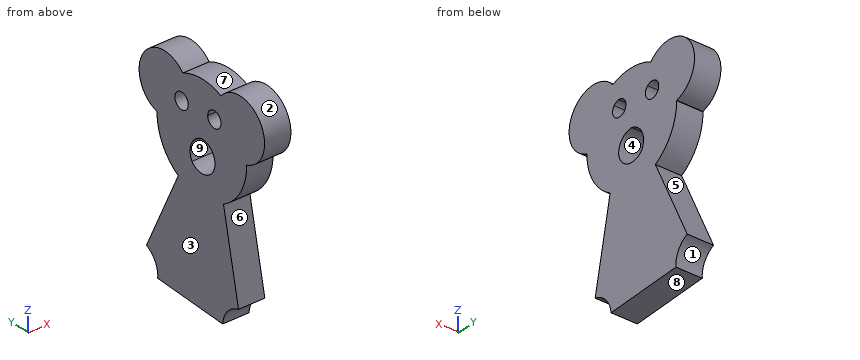
```python
from build123d import *

# Parameters (mm, degrees)
F1_DEPTH = 25


with BuildPart() as f1:
    # F0 (on Right) → F1 (new body)
    with BuildSketch(Plane.YZ):
        with BuildLine():
            Line((62.268494035, -117.2657224541), (26.5148173721, -42.9157082976))
            ThreePointArc((26.5148173721, -42.9157082976), (1.2487643575, -50.4304882639), (-24.3582585984, -44.1754320523))
            Line((-24.3582585984, -44.1754320523), (-41.1918519377, -124.9397814602))
            ThreePointArc((-41.1918519377, -124.9397814602), (-28.905337679, -132.0868997864), (-23.3544766233, -145.1722990748))
            Line((-23.3544766233, -145.1722990748), (49.5911414452, -139.3371221753))
            ThreePointArc((49.5911414452, -139.3371221753), (52.5088729266, -126.3365028199), (62.268494035, -117.2657224541))
        make_face()
        with BuildLine():
            ThreePointArc((26.5148173721, -42.9157082976), (44.0588165312, -24.5685621237), (50.4459469032, 0))
            ThreePointArc((50.4459469032, 0), (50.4457051903, 0.1561627636), (50.4449800541, 0.3123240306))
            ThreePointArc((50.4449800541, 0.3123240306), (48.3675580647, 14.3308368847), (42.4729821328, 27.2183641629))
            Line((42.4729821328, 27.2183641629), (27.7815824315, 27.2183641629))
            ThreePointArc((27.7815824315, 27.2183641629), (29.6215359729, 24.6926196845), (30.2725235865, 21.6363099275))
            ThreePointArc((30.2725235865, 21.6363099275), (19.7162138294, 14.7872975411), (17.7634647415, 27.2183641629))
            Line((17.7634647415, 27.2183641629), (-8.2927525458, 27.2183641629))
            ThreePointArc((-8.2927525458, 27.2183641629), (-7.0141543228, 24.9776791667), (-6.5704554783, 22.4362988324))
            ThreePointArc((-6.5704554783, 22.4362988324), (-16.6118358125, 15.379997677), (-19.8481584107, 27.2183641629))
            Line((-19.8481584107, 27.2183641629), (-42.4729821328, 27.2183641629))
            ThreePointArc((-42.4729821328, 27.2183641629), (-48.3583492389, 14.361880721), (-50.4445375277, 0.3770843017))
            ThreePointArc((-50.4445375277, 0.3770843017), (-43.5327032866, -25.4891605102), (-24.3582585984, -44.1754320523))
            ThreePointArc((-24.3582585984, -44.1754320523), (1.2487643575, -50.4304882639), (26.5148173721, -42.9157082976))
        make_face()
        with BuildLine():
            ThreePointArc((11.1447488889, -24.0004807711), (-13.3697300078, -20.7961057501), (0, 0))
            ThreePointArc((0, 0), (11.7053783119, -9.1523479333), (11.1447488889, -24.0004807711))
        make_face(mode=Mode.SUBTRACT)
        with BuildLine():
            Line((27.7815824315, 27.2183641629), (42.4729821328, 27.2183641629))
            ThreePointArc((42.4729821328, 27.2183641629), (33.2264505165, 37.9578258733), (21.3576968642, 45.7016667487))
            ThreePointArc((21.3576968642, 45.7016667487), (-0.0323808915, 50.4459365106), (-21.4163503965, 45.6742103889))
            ThreePointArc((-21.4163503965, 45.6742103889), (-33.2508085276, 37.9364902332), (-42.4729821328, 27.2183641629))
            Line((-42.4729821328, 27.2183641629), (-19.8481584107, 27.2183641629))
            ThreePointArc((-19.8481584107, 27.2183641629), (-17.5022305288, 29.105100824), (-14.6033657252, 29.9173419862))
            ThreePointArc((-14.6033657252, 29.9173419862), (-11.1212042341, 29.3320886421), (-8.2927525458, 27.2183641629))
            Line((-8.2927525458, 27.2183641629), (17.7634647415, 27.2183641629))
            ThreePointArc((17.7634647415, 27.2183641629), (22.7725235865, 29.1363099275), (27.7815824315, 27.2183641629))
        make_face()
        with BuildLine():
            ThreePointArc((-42.4729821328, 27.2183641629), (-33.2508085276, 37.9364902332), (-21.4163503965, 45.6742103889))
            ThreePointArc((-21.4163503965, 45.6742103889), (-66.0475916451, 42.3259048742), (-50.4445375277, 0.3770843017))
            ThreePointArc((-50.4445375277, 0.3770843017), (-48.3583492389, 14.361880721), (-42.4729821328, 27.2183641629))
        make_face()
        with BuildLine():
            ThreePointArc((42.4729821328, 27.2183641629), (48.3675580647, 14.3308368847), (50.4449800541, 0.3123240306))
            ThreePointArc((50.4449800541, 0.3123240306), (66.0999711215, 42.3594717111), (21.3576968642, 45.7016667487))
            ThreePointArc((21.3576968642, 45.7016667487), (33.2264505165, 37.9578258733), (42.4729821328, 27.2183641629))
        make_face()
    extrude(amount=F1_DEPTH)


solid = f1.part
```
CAD build for the part. Positions are in the model's coordinates, mm. Face numbers are marked on the shaded views. A direction names the side the tool comes from. Coordinates: 2 decimals unless noted, no trailing zeros. Order: outer loops, then holes, each group sorted by start corner. A loop starts at its lowest first (then second) coordinate and runs counter-clockwise, first axis right, second up. Notation, with made-up numbers: M 11.5,50.5 L 39.5,50.5 A25 cw 39.5,68.5 Z; hole C -37.75,30.5 d3. An arc over 180 degrees is marked long. Write each question's results on one line, items separated by ' | '. Start each with the question number.
Q1. Pull direction Y, two halves, no side cores. Call the marked faces 1, 2, 3 and 4: +Y half, -Y half, draft (parallel to the pull), parting line (faces both ways), or undercut.
Q2. Cut at D-D (z = -102). List the corners of the cut face in (x, y), then the cut area to 3 significant figures.
Q3. Flat gauge pins, fed straight in: P1, Ø2, axis at x = 12, y = 24.5, coming from the -Z side; P2, Ø5, axis at x = 20, y = 8, coming from the -Z side; P3, Ø6, axis at x = 3.5, z = -107, coming from the -Y side. Where does each tip first touch, or does it go through?
Q4. Cut at B-B (x = 17.75). List the corners of the cut face in (y, z), then the cut area to 3 significant figures.
Q5. Drill centre lines: probe 1 along Y at (x, z) = (8, 17.5); probe 2 along Z at (x, y) = (14.5, -18); probe 3 along Z at (x, y) = (19, 23.5). Where is each one in solid material? Low to high. Write a range as from..to.
Q6. Cut at A-A (y = -31). List the corners of the cut face in (x, z).
Q7. Which spindle directions (+Z, -Z, +X, -X, +Y, -Y) get a long thin tool onto all of the face, cutting with end or side? Do the marked faces 5, 6, 7, 8 and 9. Say none if no direction does.
Q8. Cut at C-C (y = 6). List the corners of the cut face in (x, z), then the cut area to 3 significant figures.
Found:
1) face 1: +Y half | face 2: undercut | face 3: draft | face 4: undercut
2) outline: M 0,-36.41 L 25,-36.41 L 25,54.93 L 0,54.93 Z | area: 2,280 mm²
3) P1: z = -141.42 | P2: z = -142.86 | P3: y = -38.08
4) outline: M -50.44,0.38 A50.45 ccw -24.36,-44.18 L -41.19,-124.94 A22.5 cw -23.35,-145.17 L 49.59,-139.34 A22.5 cw 62.27,-117.27 L 26.51,-42.92 A50.45 ccw 50.45,0 A50.45 ccw 50.44,0.31 A28.06 ccw long 21.36,45.7 A50.45 ccw -21.42,45.67 A28 ccw long Z; hole C -14.07,22.44 d15; hole M 0,0 A14.63 ccw long 11.14,-24 A16.33 ccw Z; hole C 22.77,21.64 d15 | area: 17,300 mm²
5) probe 1: -68.73..-19.72, -8.42..16.52, 29.03..68.8 | probe 2: -144.74..16.05, 28.82..47.13 | probe 3: -141.42..14.17, 29.1..47.89
6) outline: M 0,-130 L 25,-130 L 25,-76.04 L 0,-76.04 Z; M 0,-39.8 L 25,-39.8 L 25,52.76 L 0,52.76 Z
7) face 5: +X, -X, +Y | face 6: +X, -X, -Y | face 7: +Z, +X, -X | face 8: -Z, +X, -X, +Y | face 9: +X, -X
8) outline: M 0,-142.82 L 25,-142.82 L 25,-27.94 L 0,-27.94 Z; M 0,-2.48 L 25,-2.48 L 25,50.09 L 0,50.09 Z | area: 4,190 mm²
